Read the model definition and answer for the solid it produces. Units are mm, in the model's axes. A direction names the side the tool comes from. Coordinates: 2 decimals unless noted, no trailing zeros. Loops run counter-clockwise (first coordinate to the right, second up) from the corner with the lowest first, then second, coordinate; pieces in that order, holes last. Notation, with made-up numbers: (44.5, 15.25) -> (51.5, 15.25) arc R19 cw to (51.5, 36.25) -> close; hole circle Ø4 at (-28.75, 82.5). An arc over 180 degrees is marked (long way). Answer as a JSON object with one key per item and string values. Group by question number.
Q1. The part is cut by section C-C on z = 80. Write down the section's boundary in (x, y).
Q2. The part is cut by section B-B on y = -21. Write down the section's boundary in (x, z), and give its area (3 significant figures).
Q3. For faces 4 (the flat face through (0, -59, -74)), 5 (the flat face through (15.96, -82.66, -80.99)), 6 (the flat face through (0, -84.619, -80)), 7 (the flat face through (0, -84, 84.075)), 8 (the cylindrical face through (22.134, -80.878, 82.751)), determine the directions among +Z, -Z, +X, -X, +Y, -Y from which every point of the face is accessible in a straight line to the end or side of a thin tool.
Q4. The part is cut by section A-A on z = -43. Write down the section's boundary in (x, y), and give its area (3 significant figures).
Q5. Straight lines are drawn through the part: line 1 along Z through (x, y) = (-18, -77.75); line 2 along X through (y, z) = (-85, -80); line 3 along Z through (x, y) = (0, -2.25). For each, find the intervals that lie inside material, in ascending order. Write a range as [from, to].
Q6. Each of these flat-tipped pins is pushed along its axis until it touches: P1, Ø6, axis at x = 3, z = 10.5, coming from the -Y side; P2, Ø5, axis at x = -18, z = -80, coming from the -Y side; P3, Ø6, axis at x = -11, z = 69, coming from the +Y side; P4, Ø7.5, axis at x = 18, z = 80, coming from the +Y side. Where does it stop, or does it pass through?
Q7. The part is cut by section D-D on x = 18. Write down the section's boundary in (y, z).
Q8. Determine the mould class of faces 1 (the conical face through (-1.39, 5.73, -40.83)), 2 (the flat face through (-6.857, -88.615, -80.084)), 3 (the flat face through (0, -53, -86)) for opening direction Z: released by +Z, released by -Z, zero draft, split by the parting line, or undercut.
from build123d import *

# Parameters (mm, degrees)
SKETCH2_W                                       = 15
SKETCH2_H                                       = 15
BOSS_EXTRUDE1_DEPTH                             = 86
SKETCH3_W                                       = 15
SKETCH3_H                                       = 12
BOSS_EXTRUDE2_DEPTH                             = 85
BOSS_EXTRUDE3_DEPTH                             = 12
SKETCH6_R                                       = 4.75
SKETCH6_R_2                                     = 2.1
CUT_EXTRUDE1_DEPTH                              = 10
CUT_EXTRUDE1_DIRECTION_2_REACH                  = 82.16
CUT_EXTRUDE2_REACH                              = 21.84
SKETCH6_2_R                                     = 2.1
CSK_FOR_M3_OVAL_HEAD_MACHINE_SCREW1_D           = 5
CSK_FOR_M3_OVAL_HEAD_MACHINE_SCREW1_CSINK_D     = 5.4
CSK_FOR_M3_OVAL_HEAD_MACHINE_SCREW1_CSINK_ANGLE = 8
CUT_EXTRUDE4_REACH                              = 174
SKETCH8_R                                       = 7.2
CUT_EXTRUDE5_START                              = -1.925
SKETCH9_R                                       = 13.1
CUT_EXTRUDE5_DEPTH                              = 8.15
CUT_EXTRUDE6_REACH                              = 174


with BuildPart() as part:
    # Sketch2 → Boss-Extrude1 (new body)
    with BuildSketch(Plane.XY):
        Rectangle(SKETCH2_W, SKETCH2_H)
    extrude(amount=BOSS_EXTRUDE1_DEPTH)

    # Sketch3 → Boss-Extrude2 (add)
    with BuildSketch(Plane.XZ.offset(7.5)):
        with Locations((0, 80)):
            Rectangle(SKETCH3_W, SKETCH3_H)
    extrude(amount=BOSS_EXTRUDE2_DEPTH)

    # Sketch4 → Boss-Extrude3 (add)
    with BuildSketch(Plane.XY.offset(86)):
        with BuildLine():
            Line((-25, -92.5), (25, -92.5))
            ThreePointArc((25, -92.5), (0, -67.5), (-25, -92.5))
        make_face()
    extrude(amount=-BOSS_EXTRUDE3_DEPTH)

    # Sketch6 → Cut-Extrude1 (cut)
    with BuildSketch(Plane(origin=(0, -72.66, 0), x_dir=(-1, 0, 0), z_dir=(0, -1, 0))):
        with Locations((-18, -80)):
            Circle(SKETCH6_R)
        with Locations((-18, -80)):
            Circle(SKETCH6_R_2, mode=Mode.SUBTRACT)
        with Locations((18, -80)):
            Circle(SKETCH6_R)
        with Locations((18, -80)):
            Circle(SKETCH6_R_2, mode=Mode.SUBTRACT)
    extrude(amount=CUT_EXTRUDE1_DEPTH, mode=Mode.SUBTRACT)

    # Sketch6 → Cut-Extrude1 direction 2 (cut, up to next)
    with BuildSketch(Plane(origin=(0, -72.66, 0), x_dir=(-1, 0, 0), z_dir=(0, -1, 0)), mode=Mode.PRIVATE) as cut_extrude1_direction_2_sk1:
        with Locations((-18, -80)):
            Circle(SKETCH6_R)
        with Locations((-18, -80)):
            Circle(SKETCH6_R_2, mode=Mode.SUBTRACT)
    cut_extrude1_direction_2_tool1 = extrude(cut_extrude1_direction_2_sk1.sketch, amount=-CUT_EXTRUDE1_DIRECTION_2_REACH, mode=Mode.PRIVATE) & part.part
    add(cut_extrude1_direction_2_tool1.solids().sort_by_distance((22.61565, -72.66, 80))[0], mode=Mode.SUBTRACT)
    # Sketch6 → Cut-Extrude1 direction 2 (cut, up to next)
    with BuildSketch(Plane(origin=(0, -72.66, 0), x_dir=(-1, 0, 0), z_dir=(0, -1, 0)), mode=Mode.PRIVATE) as cut_extrude1_direction_2_sk2:
        with Locations((18, -80)):
            Circle(SKETCH6_R)
        with Locations((18, -80)):
            Circle(SKETCH6_R_2, mode=Mode.SUBTRACT)
    cut_extrude1_direction_2_tool2 = extrude(cut_extrude1_direction_2_sk2.sketch, amount=-CUT_EXTRUDE1_DIRECTION_2_REACH, mode=Mode.PRIVATE) & part.part
    add(cut_extrude1_direction_2_tool2.solids().sort_by_distance((-13.38435, -72.66, 80))[0], mode=Mode.SUBTRACT)

    # Sketch6<2> → Cut-Extrude2 (cut, up to next)
    with BuildSketch(Plane(origin=(0, -72.66, 0), x_dir=(-1, 0, 0), z_dir=(0, -1, 0)), mode=Mode.PRIVATE) as cut_extrude2_sk1:
        with Locations((-18, -80)):
            Circle(SKETCH6_2_R)
    cut_extrude2_tool1 = extrude(cut_extrude2_sk1.sketch, amount=CUT_EXTRUDE2_REACH, mode=Mode.PRIVATE) & part.part
    add(cut_extrude2_tool1.solids().sort_by_distance((18, -72.66, 80))[0], mode=Mode.SUBTRACT)
    # Sketch6<2> → Cut-Extrude2 (cut, up to next)
    with BuildSketch(Plane(origin=(0, -72.66, 0), x_dir=(-1, 0, 0), z_dir=(0, -1, 0)), mode=Mode.PRIVATE) as cut_extrude2_sk2:
        with Locations((18, -80)):
            Circle(SKETCH6_2_R)
    cut_extrude2_tool2 = extrude(cut_extrude2_sk2.sketch, amount=CUT_EXTRUDE2_REACH, mode=Mode.PRIVATE) & part.part
    add(cut_extrude2_tool2.solids().sort_by_distance((-18, -72.66, 80))[0], mode=Mode.SUBTRACT)

    # CSK for M3 Oval Head Machine Screw1 (through all)
    with Locations(Plane(origin=(0, 7.5, 0), x_dir=(1, 0, 0), z_dir=(0, 1, 0))):
        with Locations((0, -43)):
            CounterSinkHole(CSK_FOR_M3_OVAL_HEAD_MACHINE_SCREW1_D / 2, CSK_FOR_M3_OVAL_HEAD_MACHINE_SCREW1_CSINK_D / 2, counter_sink_angle=CSK_FOR_M3_OVAL_HEAD_MACHINE_SCREW1_CSINK_ANGLE)

    # Mirror1: part across plane


with BuildPart() as part_1:
    add(part.part)
    add(part.part.mirror(Plane.XY))

    # Sketch8 → Cut-Extrude4 (cut, up to next)
    with BuildSketch(Plane.XY.offset(86), mode=Mode.PRIVATE) as cut_extrude4_sk1:
        with Locations((0, -92.5)):
            Circle(SKETCH8_R)
    cut_extrude4_tool1 = extrude(cut_extrude4_sk1.sketch, amount=-CUT_EXTRUDE4_REACH, mode=Mode.PRIVATE) & part_1.part
    add(cut_extrude4_tool1.solids().sort_by_distance((0, -92.5, 86))[0], mode=Mode.SUBTRACT)

    # Sketch9 → Cut-Extrude5 (cut)
    with BuildSketch(Plane.XY.offset(86).offset(CUT_EXTRUDE5_START)):
        with Locations((0, -92.5)):
            Circle(SKETCH9_R)
    extrude(amount=-CUT_EXTRUDE5_DEPTH, mode=Mode.SUBTRACT)

    # Sketch10 → Cut-Extrude6 (cut, up to next)
    with BuildSketch(Plane(origin=(0, 0, -86), x_dir=(-1, 0, 0), z_dir=(0, 0, -1)), mode=Mode.PRIVATE) as cut_extrude6_sk1:
        Polygon((9.1, -92.5), (4.55, -84.619168826), (-4.55, -84.619168826), (-9.1, -92.5), (-4.55, -100.380831174), (4.55, -100.380831174), align=None)
    cut_extrude6_tool1 = extrude(cut_extrude6_sk1.sketch, amount=-CUT_EXTRUDE6_REACH, mode=Mode.PRIVATE) & part_1.part
    add(cut_extrude6_tool1.solids().sort_by_distance((0, -92.5, -86))[0], mode=Mode.SUBTRACT)


solid = part_1.part
Final values:
{
 "1": {"outline": "(-25, -92.5) -> (-20.1, -92.5) -> (-20.1, -82.66) -> (-22.75, -82.66) -> (-22.75, -82.13) arc R25 ccw to start; (-15.9, -92.5) -> (-13.1, -92.5) arc R13.1 cw to (13.1, -92.5) -> (15.9, -92.5) -> (15.9, -82.66) -> (13.25, -82.66) -> (13.25, -71.3) arc R25 ccw to (7.5, -68.65) -> (7.5, 7.5) -> (-7.5, 7.5) -> (-7.5, -68.65) arc R25 ccw to (-13.25, -71.3) -> (-13.25, -82.66) -> (-15.9, -82.66) -> close; (20.1, -92.5) -> (25, -92.5) arc R25 ccw to (22.75, -82.13) -> (22.75, -82.66) -> (20.1, -82.66) -> close"},
 "2": {"outline": "(-7.5, -86) -> (7.5, -86) -> (7.5, -74) -> (-7.5, -74) -> close; (-7.5, 74) -> (7.5, 74) -> (7.5, 86) -> (-7.5, 86) -> close", "area": "360 mm2"},
 "3": {"face 4": "+X, -X, -Y", "face 5": "+Y", "face 6": "-Z, -Y", "face 7": "-Y", "face 8": "+Z, -Z, +X, +Y"},
 "4": {"outline": "(-7.5, -7.5) -> (-2.5, -7.5) -> (-2.5, 4.64) -> (-2.7, 7.5) -> (-7.5, 7.5) -> close; (2.5, -7.5) -> (7.5, -7.5) -> (7.5, 7.5) -> (2.7, 7.5) -> (2.5, 4.64) -> close", "area": "149 mm2"},
 "5": {"line 1": "z = [-86, -84.75], [-75.25, -74], [74, 75.25], [84.75, 86]", "line 2": "x = [-23.85, -20.1], [-15.9, -4.77], [4.77, 15.9], [20.1, 23.85]", "line 3": "z = [-86, -45.5], [-40.5, 40.5], [45.5, 86]"},
 "6": {"P1": "stops at y = -7.5", "P2": "stops at y = -92.5", "P3": "passes through", "P4": "stops at y = -82.66"},
 "7": {"outline": "(-92.5, -86) -> (-75.15, -86) -> (-75.15, -84.75) -> (-82.66, -84.75) -> (-82.66, -82.1) -> (-92.5, -82.1) -> close; (-92.5, -77.9) -> (-82.66, -77.9) -> (-82.66, -75.25) -> (-75.15, -75.25) -> (-75.15, -74) -> (-92.5, -74) -> close; (-92.5, 74) -> (-75.15, 74) -> (-75.15, 75.25) -> (-82.66, 75.25) -> (-82.66, 77.9) -> (-92.5, 77.9) -> close; (-92.5, 82.1) -> (-82.66, 82.1) -> (-82.66, 84.75) -> (-75.15, 84.75) -> (-75.15, 86) -> (-92.5, 86) -> close"},
 "8": {"face 1": "undercut", "face 2": "zero draft", "face 3": "released by -Z"}
}
